Here's how the part is built. I have some questions about the finished solid (model axes, mm). Face numbers are marked on the shaded views. Coordinates: 2 decimals unless noted, no trailing zeros. Write each loop counter-clockwise with the first axis right and the second up, starting at its lowest first coordinate (ties: lowest second). Pieces come first, ordered by that corner, then holes.
(1) Imagine slicing it at B-B, the plane z = 0.9. List the corners of the cut face in (x, y) for me.
(2) Thinking about a two-plate mould opening in Y: for the marked faces 1, 2 and 3, which applies, released by +Y, released by -Y, zero draft, split by the parting line, or undercut?
(3) Imagine slicing it at D-D, the plane x = 3.5. List the corners of the cut face in (y, z) for me, plus the area to 4 significant figures.
(4) For pin 1 Ø5 at (x, y) = (-5, -1) entering from +Z; pin 2 Ø0.6 at (y, z) = (2, 2.5) entering from -X, each with a flat end and sliding along its axis, tell me the tip position at first contact or that it passes through.
(5) Imagine slicing it at A-A, the plane x = -20. List the corners of the cut face in (y, z) for me, plus the area to 3 significant figures.
(6) Please list where these lines run through material, in increasing order: probe 1 along X at (y, z) = (4.75, 1.9); probe 2 along X at (y, z) = (-2, 2.25); probe 3 along Y at (x, z) = (20, 0.8).
(7) Imagine slicing it at C-C, the plane y = -2.25. List the corners of the cut face in (x, z) for me.
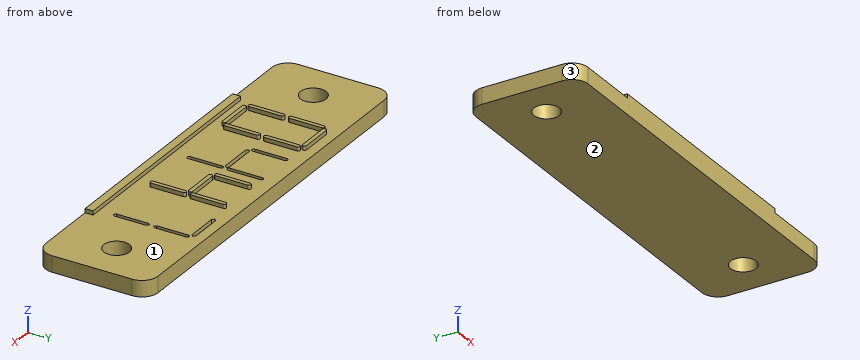
```python
from build123d import *

# Parameters (mm, degrees)
SKETCH2_W           = 50
SKETCH2_H           = 14
BOSS_EXTRUDE1_DEPTH = 2.5
SKETCH4_OUTSIDE_W   = 62.396
SKETCH4_OUTSIDE_H   = 26.396
SKETCH4_OUTSIDE_W_2 = 30
SKETCH4_OUTSIDE_H_2 = 1
CUT_EXTRUDE1_DEPTH  = 0.5
SKETCH5_R           = 1.6
CUT_EXTRUDE2_DEPTH  = 2
FILLET2_R           = 2
CUT_EXTRUDE7_DEPTH  = 0.5
BOSS_EXTRUDE4_DEPTH = 0.5


with BuildPart() as part:
    # Sketch2 → Boss-Extrude1 (new body)
    with BuildSketch(Plane.XY):
        Rectangle(SKETCH2_W, SKETCH2_H)
    extrude(amount=BOSS_EXTRUDE1_DEPTH)

    # Sketch4 outside → Cut-Extrude1 (cut)
    with BuildSketch(Plane.XY.offset(2.5)):
        Rectangle(SKETCH4_OUTSIDE_W, SKETCH4_OUTSIDE_H)
        with Locations((0, -6.5)):
            Rectangle(SKETCH4_OUTSIDE_W_2, SKETCH4_OUTSIDE_H_2, mode=Mode.SUBTRACT)
    extrude(amount=-CUT_EXTRUDE1_DEPTH, mode=Mode.SUBTRACT)

    # Sketch5 → Cut-Extrude2 (cut)
    with BuildSketch(Plane.XY.offset(2)):
        with Locations((-20, 0)):
            Circle(SKETCH5_R)
        with Locations((20, 0)):
            Circle(SKETCH5_R)
    extrude(amount=-CUT_EXTRUDE2_DEPTH, mode=Mode.SUBTRACT)

    # Fillet2
    fillet2_edges = [part.edges().sort_by_distance(p)[0] for p in [
        (25, -7, 1),
        (-25, -7, 1),
        (-25, 7, 1),
        (25, 7, 1),
    ]]
    fillet(fillet2_edges, radius=FILLET2_R)

    # Sketch6 → Cut-Extrude7 (cut)
    with BuildSketch(Plane.XY.offset(2)):
        with BuildLine():
            Line((-5.75, 0.75), (-1.75, 0.75))
            ThreePointArc((-1.75, 0.75), (-1.5, 0.5), (-1.75, 0.25))
            Line((-1.75, 0.25), (-5.75, 0.25))
            ThreePointArc((-5.75, 0.25), (-6, 0.5), (-5.75, 0.75))
        make_face()
        with BuildLine():
            Line((-6.5, 1), (-6.5, 5))
            ThreePointArc((-6.5, 5), (-6.25, 5.25), (-6, 5))
            Line((-6, 5), (-6, 1))
            ThreePointArc((-6, 1), (-6.25, 0.75), (-6.5, 1))
        make_face()
        with BuildLine():
            Line((-1, 0), (-1, -4))
            ThreePointArc((-1, -4), (-1.25, -4.25), (-1.5, -4))
            Line((-1.5, -4), (-1.5, 0))
            ThreePointArc((-1.5, 0), (-1.25, 0.25), (-1, 0))
        make_face()
        with BuildLine():
            Line((-1.5, 1), (-1.5, 5))
            ThreePointArc((-1.5, 5), (-1.25, 5.25), (-1, 5))
            Line((-1, 5), (-1, 1))
            ThreePointArc((-1, 1), (-1.25, 0.75), (-1.5, 1))
        make_face()
        Polygon((14, 0), (14, -4), (13.75, -4.25), (13.5, -4), (13.5, 0), (13.75, 0.25), align=None)
        Polygon((13.25, 5.25), (9.25, 5.25), (9, 5.5), (9.25, 5.75), (13.25, 5.75), (13.5, 5.5), align=None)
        Polygon((13.5, 1), (13.5, 5), (13.75, 5.25), (14, 5), (14, 1), (13.75, 0.75), align=None)
    extrude(amount=-CUT_EXTRUDE7_DEPTH, mode=Mode.SUBTRACT)

    # Sketch6<10> → Boss-Extrude4 (add)
    with BuildSketch(Plane.XY.offset(2)):
        with BuildLine():
            Line((-9, 1), (-9, 5))
            ThreePointArc((-9, 5), (-8.75, 5.25), (-8.5, 5))
            Line((-8.5, 5), (-8.5, 1))
            ThreePointArc((-8.5, 1), (-8.75, 0.75), (-9, 1))
        make_face()
        with BuildLine():
            Line((-13.25, -4.25), (-9.25, -4.25))
            ThreePointArc((-9.25, -4.25), (-9, -4.5), (-9.25, -4.75))
            Line((-9.25, -4.75), (-13.25, -4.75))
            ThreePointArc((-13.25, -4.75), (-13.5, -4.5), (-13.25, -4.25))
        make_face()
        with BuildLine():
            Line((-13.25, 5.75), (-9.25, 5.75))
            ThreePointArc((-9.25, 5.75), (-9, 5.5), (-9.25, 5.25))
            Line((-9.25, 5.25), (-13.25, 5.25))
            ThreePointArc((-13.25, 5.25), (-13.5, 5.5), (-13.25, 5.75))
        make_face()
        with BuildLine():
            Line((-13.5, 0), (-13.5, -4))
            ThreePointArc((-13.5, -4), (-13.75, -4.25), (-14, -4))
            Line((-14, -4), (-14, 0))
            ThreePointArc((-14, 0), (-13.75, 0.25), (-13.5, 0))
        make_face()
        with BuildLine():
            Line((-14, 1), (-14, 5))
            ThreePointArc((-14, 5), (-13.75, 5.25), (-13.5, 5))
            Line((-13.5, 5), (-13.5, 1))
            ThreePointArc((-13.5, 1), (-13.75, 0.75), (-14, 1))
        make_face()
        with BuildLine():
            Line((-8.5, 0), (-8.5, -4))
            ThreePointArc((-8.5, -4), (-8.75, -4.25), (-9, -4))
            Line((-9, -4), (-9, 0))
            ThreePointArc((-9, 0), (-8.75, 0.25), (-8.5, 0))
        make_face()
        with BuildLine():
            Line((1.5, 1), (1.5, 5))
            ThreePointArc((1.5, 5), (1.25, 5.25), (1, 5))
            Line((1, 5), (1, 1))
            ThreePointArc((1, 1), (1.25, 0.75), (1.5, 1))
        make_face()
        with BuildLine():
            Line((1.75, 0.25), (5.75, 0.25))
            ThreePointArc((5.75, 0.25), (6, 0.5), (5.75, 0.75))
            Line((5.75, 0.75), (1.75, 0.75))
            ThreePointArc((1.75, 0.75), (1.5, 0.5), (1.75, 0.25))
        make_face()
        with BuildLine():
            Line((6.5, 1), (6.5, 5))
            ThreePointArc((6.5, 5), (6.25, 5.25), (6, 5))
            Line((6, 5), (6, 1))
            ThreePointArc((6, 1), (6.25, 0.75), (6.5, 1))
        make_face()
        with BuildLine():
            Line((6.5, 0), (6.5, -4))
            ThreePointArc((6.5, -4), (6.25, -4.25), (6, -4))
            Line((6, -4), (6, 0))
            ThreePointArc((6, 0), (6.25, 0.25), (6.5, 0))
        make_face()
    extrude(amount=BOSS_EXTRUDE4_DEPTH)


solid = part.part
```
Recorded:
1. outline: (-25, -5) arc R2 ccw to (-23, -7) - (23, -7) arc R2 ccw to (25, -5) - (25, 5) arc R2 ccw to (23, 7) - (-23, 7) arc R2 ccw to (-25, 5) - close; hole circle Ø3.2 at (-20, 0); hole circle Ø3.2 at (20, 0)
2. face 1: undercut
2. face 2: zero draft
2. face 3: released by -Y
3. outline: (-7, 0) - (7, 0) - (7, 2) - (0.75, 2) - (0.75, 2.5) - (0.25, 2.5) - (0.25, 2) - (-6, 2) - (-6, 2.5) - (-7, 2.5) - close
3. area: 28.75 mm2
4. pin 1: stops at z = 2
4. pin 2: stops at x = -14
5. outline: (-7, 0) - (-1.6, 0) - (-1.6, 2) - (-7, 2) - close; (1.6, 0) - (7, 0) - (7, 2) - (1.6, 2) - close
5. area: 21.6 mm2
6. probe 1: x = -25 to -6.5, -6 to -1.5, -1 to 13.5, 14 to 25
6. probe 2: x = -14 to -13.5, -9 to -8.5, 6 to 6.5
6. probe 3: y = -7 to -1.6, 1.6 to 7
7. outline: (-25, 0) - (25, 0) - (25, 2) - (14, 2) - (14, 1.5) - (13.5, 1.5) - (13.5, 2) - (6.5, 2) - (6.5, 2.5) - (6, 2.5) - (6, 2) - (-1, 2) - (-1, 1.5) - (-1.5, 1.5) - (-1.5, 2) - (-8.5, 2) - (-8.5, 2.5) - (-9, 2.5) - (-9, 2) - (-13.5, 2) - (-13.5, 2.5) - (-14, 2.5) - (-14, 2) - (-25, 2) - close
